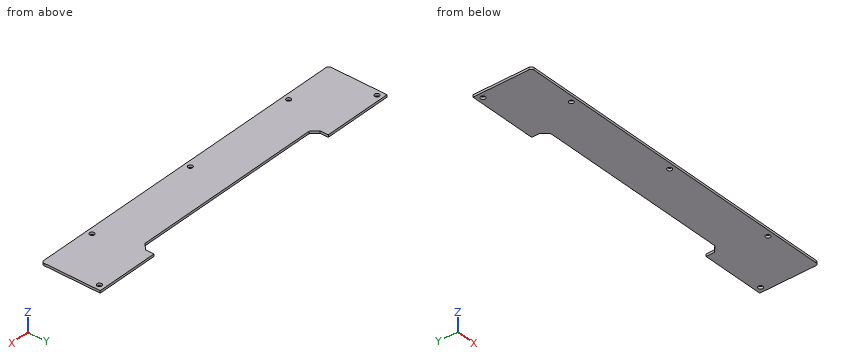
```python
from build123d import *

# Parameters (mm, degrees)
F0_W     = 248.269176
F0_H     = 43.005985
F0_R     = 1.7272
F1_DEPTH = 1.70942
F2_R     = 1.98374
F3_W     = 150.955984
F3_H     = 10.467619
F4_DEPTH = 1.70942
F5_SIZE  = 4.415511


with BuildPart() as f1:
    # F0 (on Top) → F1 (new body)
    with BuildSketch(Plane.XY):
        with Locations((124.134588, -21.502992)):
            Rectangle(F0_W, F0_H)
        with Locations((39.037235, -39.037235)):
            Circle(F0_R, mode=Mode.SUBTRACT)
        with Locations((124.134588, -39.037235)):
            Circle(F0_R, mode=Mode.SUBTRACT)
        with Locations((209.231941, -39.037235)):
            Circle(F0_R, mode=Mode.SUBTRACT)
        with Locations((3.96875, -3.96875)):
            Circle(F0_R, mode=Mode.SUBTRACT)
        with Locations((244.300426, -3.96875)):
            Circle(F0_R, mode=Mode.SUBTRACT)
    extrude(amount=F1_DEPTH)

    # F2
    f2_edges = [f1.edges().sort_by_distance(p)[0] for p in [
        (0, -43.005985, 0.85471),
        (248.269176, -43.005985, 0.85471),
    ]]
    fillet(f2_edges, radius=F2_R)

    # F3 (on face) → F4 (cut, through all)
    with BuildSketch(Plane.XY.offset(1.70942)):
        with Locations((126.261038, -5.233809)):
            Rectangle(F3_W, F3_H)
    extrude(amount=-F4_DEPTH, mode=Mode.SUBTRACT)

    # F5
    f5_edges = [f1.edges().sort_by_distance(p)[0] for p in [
        (50.783046, -10.467619, 0.85471),
        (201.73903, -10.467619, 0.85471),
    ]]
    chamfer(f5_edges, length=F5_SIZE)


solid = f1.part
```
Read the model definition and answer for the solid it produces. Units are mm, in the model's axes. Give positions to 0.01 mm unless a question says otherwise; leave off trailing zeros. Write each loop counter-clockwise with the first axis right and the second up, starting at its lowest first coordinate (ties: lowest second). Pieces come first, ordered by that corner, then holes. Notation, with made-up numbers: (-2.75, 89) - (35.25, 89) arc R18 ccw to (35.25, 110) - close; hole circle Ø8 at (-39, -18). An arc over 180 degrees is marked (long way). Write item = value, one per line. Start each with the question number.
Item 1: This flat-tipped pin is pushed along its axis until it touches: P1, Ø2, axis at x = 244.3, y = -3.97, coming from the -Z side. Where does it stop, or does it pass through?
Item 2: Find section B-B (x = 110). Give the vertices of the cut face in (y, z), then the cut area to 3 significant figures.
Item 3: Find the intervals of material crossed by probe 1 along X at (y, z) = (-5, 1.6); probe 2 along Y at (x, z) = (156.5, 0.2); probe 3 along X at (y, z) = (-3, 0.2), in increasing order. Write a range as [from, to].
Item 4: Find section A-A (z = 1.1). Give the vertices of the cut face in (x, y).
Response:
q1.P1 = through
q2.outline = (-43.01, 0) - (-10.47, 0) - (-10.47, 1.71) - (-43.01, 1.71) - close
q2.area = 55.6 mm²
q3.probe_1 = [0, 2.58], [5.35, 50.78], [201.74, 242.91], [245.69, 248.27]
q3.probe_2 = [-43.01, -10.47]
q3.probe_3 = [0, 2.54], [5.4, 50.78], [201.74, 242.87], [245.73, 248.27]
q4.outline = (0, -41.02) arc R1.98 ccw to (1.98, -43.01) - (246.29, -43.01) arc R1.98 ccw to (248.27, -41.02) - (248.27, 0) - (201.74, 0) - (201.74, -6.05) - (197.32, -10.47) - (55.2, -10.47) - (50.78, -6.05) - (50.78, 0) - (0, 0) - close; hole circle Ø3.45 at (3.97, -3.97); hole circle Ø3.45 at (39.04, -39.04); hole circle Ø3.45 at (124.13, -39.04); hole circle Ø3.45 at (209.23, -39.04); hole circle Ø3.45 at (244.3, -3.97)
